Model file for the job. Use its own axes, mm. Round coordinates to 2 decimals unless told otherwise and drop trailing zeros. Order: outer loops, then holes, each group sorted by start corner. A loop starts at its lowest first (then second) coordinate and runs counter-clockwise, first axis right, second up. Notation, with made-up numbers: (-36, 32.25) - (6, 32.25) arc R22 ccw to (6, 69.25) - close; hole circle Ø1 at (-38.5, 59.5). An arc over 180 degrees is marked (long way). Write item = value, one per line.
```python
from build123d import *

# Parameters (mm, degrees)
F0_R     = 2
F0_R_2   = 1
F1_DEPTH = 10
F2_R     = 7.5
F3_DEPTH = 5
F4_R     = 1
F5_DEPTH = 15.001
F6_R     = 4


with BuildPart() as f1:
    # F0 (on Front) → F1 (new body)
    with BuildSketch(Plane.XZ):
        Circle(F0_R)
        Circle(F0_R_2, mode=Mode.SUBTRACT)
    extrude(amount=F1_DEPTH)

    # F2 (on Front) → F3 (join)
    with BuildSketch(Plane.XZ):
        Circle(F2_R)
    extrude(amount=-F3_DEPTH)

    # F4 (on face) → F5 (cut, through all)
    with BuildSketch(Plane(origin=(0, 5, 0), x_dir=(-1, 0, 0), z_dir=(0, 1, 0))):
        Circle(F4_R)
    extrude(amount=-F5_DEPTH, mode=Mode.SUBTRACT)

    # F6
    f6_edges = [f1.edges().sort_by_distance(p)[0] for p in [
        (-7.5, 5, 0),
    ]]
    fillet(f6_edges, radius=F6_R)


solid = f1.part
```
1) Mould opens along X. For faces 1 (the face through (2, 0, -2)), 2 (the face through (0, -2, -1)), 3 (the face through (0, -5, -2)) say: +X half, -X half, draft (parallel to the pull), parting line (faces both ways), or undercut.
Conclusion:
face_1 = draft
face_2 = undercut
face_3 = parting line
2) Flat gauge pins, fed straight in: pin 1 Ø1.5 at (y, z) = (-1, -1) entering from -X; pin 2 Ø2 at (y, z) = (-1.5, 1) entering from +X; pin 3 Ø4 at (x, y) = (-0.5, -4.5) entering from +Z. Where does each tip first touch, or does it go through?
Conclusion:
pin_1 = -1.98
pin_2 = 2
pin_3 = 2
3) Wall check: line 1 along Z through (x, y) = (0, -4); line 2 along Y through (x, z) = (-2.5, -2.5); line 3 along X through (y, z) = (2, 0). Give the ranges that are in metal, low to high.
Conclusion:
line_1 = -2 to -1, 1 to 2
line_2 = 0 to 5
line_3 = -7.37 to -1, 1 to 7.37
4) Cut at A-A (y = -0.5). Write the cut outline in (x, z), and give its area (3 significant figures).
Conclusion:
outline = circle Ø4 at (0, 0); hole circle Ø2 at (0, 0)
area = 9.42 mm^2
